```python
from build123d import *

# Parameters (mm, degrees)
SKETCH1_R           = 18.5
SKETCH1_R_2         = 1.75
BOSS_EXTRUDE1_DEPTH = 4.5
SKETCH2_R           = 6.4
SKETCH2_R_2         = 1.75
BOSS_EXTRUDE2_DEPTH = 3
SKETCH3_R           = 3
CUT_EXTRUDE1_DEPTH  = 2.5


with BuildPart() as part:
    # Sketch1 → Boss-Extrude1 (new body)
    with BuildSketch(Plane.XY):
        Polygon((-12.327463607, 17.616562478), (-12.327463607, -18.183437522), (-9.095169285, -21.415731844), (26.704830715, -21.415731844), (29.937125036, -18.183437522), (29.937125036, 17.616562478), (26.704830715, 20.848856799), (-9.095169285, 20.848856799), align=None)
        with Locations((8.804830715, -0.283437522)):
            Circle(SKETCH1_R, mode=Mode.SUBTRACT)
        with Locations((-6.945169285, 15.466562478)):
            Circle(SKETCH1_R_2, mode=Mode.SUBTRACT)
        with Locations((-6.945169285, -16.033437522)):
            Circle(SKETCH1_R_2, mode=Mode.SUBTRACT)
        with Locations((24.554830715, -16.033437522)):
            Circle(SKETCH1_R_2, mode=Mode.SUBTRACT)
        with Locations((24.554830715, 15.466562478)):
            Circle(SKETCH1_R_2, mode=Mode.SUBTRACT)
    extrude(amount=BOSS_EXTRUDE1_DEPTH)

    # Sketch2 → Boss-Extrude2 (add)
    with BuildSketch(Plane.XY.offset(4.5)):
        Polygon((-12.327463607, 17.616562478), (-9.095169285, 20.848856799), (26.704830715, 20.848856799), (29.937125036, 17.616562478), (29.937125036, -18.183437522), (26.704830715, -21.415731844), (-9.095169285, -21.415731844), (-12.327463607, -18.183437522), align=None)
        with Locations((8.804830715, -0.283437522)):
            Circle(SKETCH2_R, mode=Mode.SUBTRACT)
        with Locations((-6.945169285, 15.466562478)):
            Circle(SKETCH2_R_2, mode=Mode.SUBTRACT)
        with Locations((24.554830715, 15.466562478)):
            Circle(SKETCH2_R_2, mode=Mode.SUBTRACT)
        with Locations((24.554830715, -16.033437522)):
            Circle(SKETCH2_R_2, mode=Mode.SUBTRACT)
        with Locations((-6.945169285, -16.033437522)):
            Circle(SKETCH2_R_2, mode=Mode.SUBTRACT)
    extrude(amount=BOSS_EXTRUDE2_DEPTH)

    # Sketch3 → Cut-Extrude1 (cut)
    with BuildSketch(Plane.XY.offset(7.5)):
        with Locations((-6.945169285, 15.466562478)):
            Circle(SKETCH3_R)
        with Locations((24.554830715, -16.033437522)):
            Circle(SKETCH3_R)
    extrude(amount=-CUT_EXTRUDE1_DEPTH, mode=Mode.SUBTRACT)


solid = part.part
```
Here's how the part is built. I have some questions about the finished solid (model axes, mm). A direction names the side the tool comes from. Round coordinates to 2 decimals unless told otherwise and drop trailing zeros. Order: outer loops, then holes, each group sorted by start corner. A loop starts at its lowest first (then second) coordinate and runs counter-clockwise, first axis right, second up. Notation, with made-up numbers: M 8,52 L 18,52 A10 ccw 18,64 Z; hole C -15,-28 d5. An arc over 180 degrees is marked long. Answer as CSV lines item,"result".
Item 1: Imagine slicing it at A-A on y = 0.5. List the corners of the cut face in (x, z) for me.
From the geometry:
outline,"M -12.33,0 L -9.68,0 L -9.68,4.5 L 2.45,4.5 L 2.45,7.5 L -12.33,7.5 Z; M 15.16,4.5 L 27.29,4.5 L 27.29,0 L 29.94,0 L 29.94,7.5 L 15.16,7.5 Z"
Item 2: Imagine slicing it at B-B on x = -7.5. List the corners of the cut face in (y, z) for me.
From the geometry:
outline,"M -21.42,0 L -17.69,0 L -17.69,7.5 L -21.42,7.5 Z; M -14.37,0 L -9.02,0 L -9.02,4.5 L 8.46,4.5 L 8.46,0 L 13.81,0 L 13.81,5 L 12.52,5 L 12.52,7.5 L -14.37,7.5 Z; M 17.13,0 L 20.85,0 L 20.85,7.5 L 18.41,7.5 L 18.41,5 L 17.13,5 Z"
Item 3: We'd pull the mould along X, two halves only. Please class faces 1 (the cylindrical face through (23.166, -17.098, 2.465)), 2 (the flat face through (-10.734, 19.21, 3.698)), 3 (the flat face through (28.298, 19.255, 3.698)): +X half, -X half, draft (parallel to the pull), parting line (faces both ways), or undercut.
From the geometry:
face 1,"undercut"
face 2,"-X half"
face 3,"+X half"
Item 4: Which directions (+Z, -Z, +X, -X, +Y, -Y) give clear straight access to the entire face, cutting with the end or side of a thin tool? Please do faces 4 (the flat face through (-10.69, -19.82, 3.7)), 5 (the flat face through (-5, 16, 5)), 6 (the flat face through (9, -8, 4.5)).
From the geometry:
face 4,"+Z, -Z, -X, -Y"
face 5,"+Z"
face 6,"-Z"
Item 5: For pin 1 (4.5 mm diameter, centred on x = -6.95, y = 15.47, fed in from +Z); pin 2 (18.5 mm diameter, centred on x = 16, y = 5, fed in from -Z), each with a flat end and sliding along its axis, tell me the tip position at first contact or that it passes through.
From the geometry:
pin 1,"z = 5"
pin 2,"z = 4.5"
Item 6: Imagine slicing it at D-D on x = 14. List the corners of the cut face in (y, z) for me.
From the geometry:
outline,"M -21.42,0 L -18.04,0 L -18.04,4.5 L -4.02,4.5 L -4.02,7.5 L -21.42,7.5 Z; M 3.45,4.5 L 17.47,4.5 L 17.47,0 L 20.85,0 L 20.85,7.5 L 3.45,7.5 Z"
Item 7: Please list where these lines run through material, in increasing order: L1, parallel to Y at x = -8, z = 1.75; L2, parallel to Y at x = 25, z = 2; L3, parallel to X at y = -16, z = 2.75. Write a range as [from, to].
From the geometry:
L1,"[-21.42, -17.43], [-14.64, -8.02], [7.45, 14.07], [16.86, 20.85]"
L2,"[-21.42, -17.73], [-14.34, -9.23], [8.66, 13.77], [17.16, 20.85]"
L3,"[-12.33, -8.69], [-5.2, -0.95], [18.56, 22.81], [26.3, 29.94]"
Item 8: Imagine slicing it at C-C on z = 6.25. List the corners of the cut face in (x, y) for me, and give its area (3 significant figures).
From the geometry:
outline,"M -12.33,-18.18 L -9.1,-21.42 L 26.7,-21.42 L 29.94,-18.18 L 29.94,17.62 L 26.7,20.85 L -9.1,20.85 L -12.33,17.62 Z; hole C -6.95,15.47 d6; hole C -6.95,-16.03 d3.5; hole C 8.8,-0.28 d12.8; hole C 24.55,-16.03 d6; hole C 24.55,15.47 d3.5"
area,"1,560 mm2"
